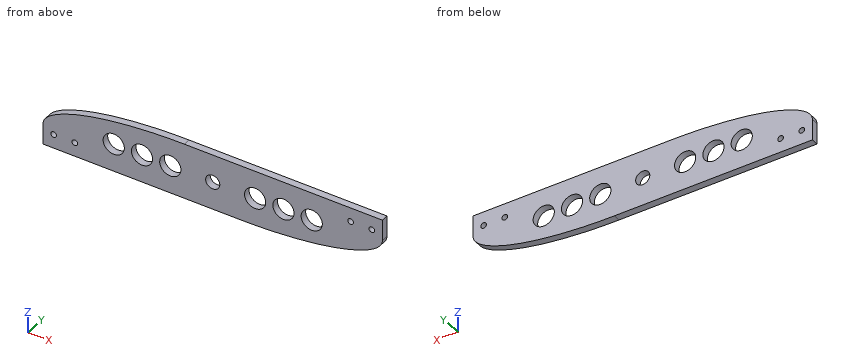
from build123d import *

# Parameters (mm, degrees)
SKETCH2_W           = 304.8
SKETCH2_H           = 50.8
SKETCH2_R           = 6.35
SKETCH2_R_2         = 9.525
SKETCH2_R_3         = 2.5527
BOSS_EXTRUDE2_DEPTH = 3.175
FILLET1_SIZE        = 127
FILLET1_SIZE_2      = 31.75


with BuildPart() as part:
    # Sketch2 → Boss-Extrude2 (new, symmetric)
    with BuildSketch(Plane(origin=(0, 0, 0), x_dir=(1, 0, 0), z_dir=(0, 1, 0))):
        Rectangle(SKETCH2_W, SKETCH2_H)
        with Locations(Location((0, 0, 0), (0, 0, 270))):
            Circle(SKETCH2_R, mode=Mode.SUBTRACT)
        with Locations(Location((-38.1, 0, 0), (0, 0, 270))):
            Circle(SKETCH2_R_2, mode=Mode.SUBTRACT)
        with Locations(Location((-63.5, 0, 0), (0, 0, 270))):
            Circle(SKETCH2_R_2, mode=Mode.SUBTRACT)
        with Locations(Location((-88.9, 0, 0), (0, 0, 270))):
            Circle(SKETCH2_R_2, mode=Mode.SUBTRACT)
        with Locations(Location((38.1, 0, 0), (0, 0, 90))):
            Circle(SKETCH2_R_2, mode=Mode.SUBTRACT)
        with Locations(Location((63.5, 0, 0), (0, 0, 90))):
            Circle(SKETCH2_R_2, mode=Mode.SUBTRACT)
        with Locations(Location((88.9, 0, 0), (0, 0, 90))):
            Circle(SKETCH2_R_2, mode=Mode.SUBTRACT)
        with Locations(Location((142.875, -12.7, 0), (0, 0, 270))):
            Circle(SKETCH2_R_3, mode=Mode.SUBTRACT)
        with Locations(Location((123.825, -12.7, 0), (0, 0, 270))):
            Circle(SKETCH2_R_3, mode=Mode.SUBTRACT)
        with Locations(Location((-142.875, 12.7, 0), (0, 0, 270))):
            Circle(SKETCH2_R_3, mode=Mode.SUBTRACT)
        with Locations(Location((-123.825, 12.7, 0), (0, 0, 270))):
            Circle(SKETCH2_R_3, mode=Mode.SUBTRACT)
    extrude(amount=BOSS_EXTRUDE2_DEPTH, both=True)

    # Fillet1
    # an asymmetric fillet: 127, 31.75 mm, written as the material it takes off along each edge
    with BuildSketch(Plane(origin=(152.4, -320.675, -25.4), x_dir=(-1, 0, 0), z_dir=(0, 1, 0))) as fillet1_piece_1:
        with BuildLine():
            Bezier((FILLET1_SIZE, 0), (0, 0), (0, FILLET1_SIZE_2), weights=[1, 0.707106781, 1])
            Line((0, FILLET1_SIZE_2), (0, 0))
            Line((0, 0), (FILLET1_SIZE, 0))
        make_face()
    extrude(amount=641.35, mode=Mode.SUBTRACT)
    with BuildSketch(Plane(origin=(-152.4, 320.675, 25.4), x_dir=(1, 0, 0), z_dir=(0, -1, 0))) as fillet1_piece_2:
        with BuildLine():
            Bezier((FILLET1_SIZE, 0), (0, 0), (0, -FILLET1_SIZE_2), weights=[1, 0.707106781, 1])
            Line((0, -FILLET1_SIZE_2), (0, 0))
            Line((0, 0), (FILLET1_SIZE, 0))
        make_face()
    extrude(amount=641.35, mode=Mode.SUBTRACT)


solid = part.part
Design review of the part built by this model. Coordinates are the model's own, in mm. Coordinates: 2 decimals unless noted, no trailing zeros. Use CSV: the item, a comma, the result in double quotes. Start each with the question number.
1. To check wall thickness, follow probe 1 along Z at (x, y) = (-135.5, 0); probe 2 along Z at (x, y) = (63.5, -0.5) (3 decimals); probe 3 along Z at (x, y) = (-89, -1.75). State the ranges of each line that lie inside material, in increasing order.
2. Add section A-A on z = -12.7. Count the separate pieces of the cut face and the enclosed holes in it, plus the area to 3 significant figures.
3. Clearance check with flat-ended pins moving along their axes: pin 1 (1 mm diameter, centred on y = 2, z = 6.5, fed in from -X); pin 2 (1 mm diameter, centred on x = 121, y = -1.5, fed in from -Z). State where each tip first meets the part, or that it passes through.
Resolved:
1,probe 1,"-25.4 to 9.48"
1,probe 2,"-23.938 to -9.525, 9.525 to 25.4"
1,probe 3,"-25.4 to -9.52, 9.52 to 21.13"
2,separate pieces,"3"
2,enclosed holes,"0"
2,area,"1,710 mm2"
3,pin 1,"x = -142.4"
3,pin 2,"z = -14.69"
